Read the model definition and answer for the solid it produces. Units are mm, in the model's axes. Round coordinates to 2 decimals unless told otherwise and drop trailing zeros.
from build123d import *

# Parameters (mm, degrees)
SKETCH1_R      = 12.7
EXTRUDE1_DEPTH = 800.79215
SKETCH2_R      = 9.5123
EXTRUDE2_DEPTH = 828.294
SKETCH3_W      = 6.35
SKETCH3_H      = 0.79375
SKETCH4_R      = 2.38125
EXTRUDE3_DEPTH = 19.05
CHAMFER1_SIZE  = 0.762


with BuildPart() as part:
    # Sketch1 → Extrude1 (new, symmetric)
    with BuildSketch(Plane(origin=(0, 0, 0), x_dir=(0, 0, -1), z_dir=(1, 0, 0))):
        Circle(SKETCH1_R)
    extrude(amount=EXTRUDE1_DEPTH, both=True)

    # Sketch2 → Extrude2 (add, symmetric)
    with BuildSketch(Plane(origin=(0, 0, 0), x_dir=(0, 0, -1), z_dir=(1, 0, 0))):
        Circle(SKETCH2_R)
    extrude(amount=EXTRUDE2_DEPTH, both=True)

    # Sketch3 → Cut-Revolve1 (revolve, cut)
    with BuildSketch(Plane.XY, mode=Mode.PRIVATE) as cut_revolve1_sk:
        with Locations((-712.4065, 12.303125)):
            Rectangle(SKETCH3_W, SKETCH3_H)
        with Locations((712.4065, 12.303125)):
            Rectangle(SKETCH3_W, SKETCH3_H)
    revolve(cut_revolve1_sk.sketch.rotate(Axis((800.79215, 0, 0), (-1, 0, 0)), 90), axis=Axis((800.79215, 0, 0), (-1, 0, 0)), mode=Mode.SUBTRACT)

    # Sketch4 → Extrude3 (cut, symmetric)
    with BuildSketch(Plane(origin=(0, 0, 0), x_dir=(1, 0, 0), z_dir=(0, 1, 0))):
        with Locations(Location((-689.5973, 0, 0), (0, 0, 270))):
            Circle(SKETCH4_R)
        with Locations(Location((689.5973, 0, 0), (0, 0, 270))):
            Circle(SKETCH4_R)
    extrude(amount=EXTRUDE3_DEPTH, both=True, mode=Mode.SUBTRACT)

    # Chamfer1
    chamfer1_edges = [part.edges().sort_by_distance(p)[0] for p in [
        (-828.294, 0, 9.5123),
        (828.294, 0, 9.5123),
    ]]
    chamfer(chamfer1_edges, length=CHAMFER1_SIZE)


solid = part.part
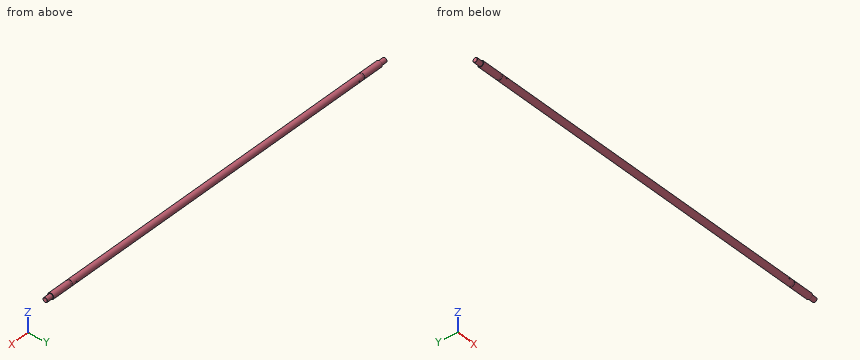
Q1. Straight lines are drawn through the part: probe 1 along X at (y, z) = (7.75, -9.25); probe 2 along X at (y, z) = (-7, -1.75); probe 3 along Y at (x, z) = (401, 4.5). For each, find the intervals that lie inside material, in ascending order.
Outcome:
probe 1: x = -800.79 to -715.58, -709.23 to 709.23, 715.58 to 800.79
probe 2: x = -828.29 to -691.21, -687.98 to 687.98, 691.21 to 828.29
probe 3: y = -11.88 to 11.88
Q2. A cutting plane is placed at A-A, the plane y = 4. Give the number of separate pieces and of enclosed holes in the cut face, plus the area to 3 significant figures.
Outcome:
separate pieces: 1
enclosed holes: 2
area: 39,500 mm2
Q3. Flat-ended cylindrical pins translate along their axes: pin 1 (4 mm diameter, centred on x = -465.5, z = 1.5, fed in from +Y); pin 2 (8 mm diameter, centred on x = -443.5, z = -10, fed in from +Y); pin 3 (10 mm diameter, centred on x = 149.5, y = -9.5, fed in from -Z); pin 4 (1 mm diameter, centred on x = -184, y = 3.5, fed in from +Z). Find the tip coordinate at first contact, or state that the pin passes through.
Outcome:
pin 1: stops at y = 12.7
pin 2: stops at y = 11.19
pin 3: stops at z = -11.88
pin 4: stops at z = 12.34
